The model under review builds one solid part; all positions refer to its coordinate system, in mm. A direction names the side the tool comes from. Give positions to 0.01 mm unless a question says otherwise; leave off trailing zeros. Loops run counter-clockwise (first coordinate to the right, second up) from the corner with the lowest first, then second, coordinate; pieces in that order, holes last. Notation, with made-up numbers: M 82.25,-21.75 L 103.25,-21.75 A6 cw 103.25,-12.75 Z; hole C 50,5 d4. An arc over 180 degrees is marked long. Put each result on its own line as item: value. Start each with the question number.
Autodesk Fusion 360 part; units mm, degrees
sketch "Sketch4" plane through (0, 0, 0) normal (0, 0, 1) x (1, 0, 0)
  circle A0 centre (0, 0) radius 25 construction
  dimension "d8" = 50
sketch "Sketch6" plane through (0, 0, 0) normal (1, 0, 0) x (0, 1, 0)
  line L0 (0, 0) -> (25, 0) construction
  line L1 (25, 0) -> (25, 10)
  line L2 (0, 0) -> (14.8, 0) construction
  line L3 (14.8, 0) -> (14.8, 10) construction
  line L4 (14.8, 10) -> (25, 10) construction
  line L5 (25, 10) -> (11.5, 10) construction
  line L6 (14.8, 0) -> (13.3946, 10) construction
  line L7 (14.8, 0) -> (24.8983, 0) construction
  line L8 (25, 10) -> (13.3946, 10)
  line L9 (13.3946, 10) -> (14.8, 0)
  line L10 (25, 0) -> (14.8, 0)
  dimension "d9" = 25
  dimension "d10" = 10
  dimension "d11" = 14.8
  dimension "d12" = 98
revolve "Revolve1" add sketch "Sketch6" angle 360 about axis through (0, 0, 1.75) along (0, 0, 1)
sketch "Sketch7" plane through (0, 0, 0) normal (0, 0, -1) x (1, 0, 0)
  circle A0 centre (0, 0) radius 25
  circle A1 centre (0, 0) radius 14.8
extrude "Extrude3" add 1 faces at (1.9773, 21.4518, 0) along direction (0, 0, -1) blind 10
sketch "Sketch8" plane through (0, 0, -10) normal (0, 0, -1) x (1, 0, 0)
  circle A0 centre (0, 0) radius 25
  circle A1 centre (0, 0) radius 14.8
  circle A2 centre (0, 0) radius 14.8
  circle A3 centre (0, 0) radius 25
  line L0 (1.5, 14.7238) -> (1.5, 24.955)
  line L1 (-1.5, 14.7238) -> (-1.5, 24.955)
  line L2 (-14.7238, 1.5) -> (-24.955, 1.5)
  line L3 (-14.7238, -1.5) -> (-24.955, -1.5)
  line L4 (-1.5, -14.7238) -> (-1.5, -24.955)
  line L5 (1.5, -14.7238) -> (1.5, -24.955)
  line L6 (14.7238, -1.5) -> (24.955, -1.5)
  line L7 (14.7238, 1.5) -> (24.955, 1.5)
  dimension "d19" = 360
extrude "Extrude4" add sketch "Sketch8" along normal blind 15 contours A0 A1 A2 A3 L0 L7 | A0 A1 A2 A3 L5 L6 | A0 A1 A2 A3 L1 L2 | A0 A1 A2 A3 L3 L4
Item 1: Consider section C-C, the plane x = 20. Write out the cut boundary in (y, z).
Item 2: Consider section A-A, the plane x = 0. Write out the cut boundary in (y, z).
Item 3: Draft analysis for pull direction X (two halves, no side actions). For faces 4 (the flat face through (11, 11, 10)), 5 (the flat face through (0, -20, -10)), 6 (the flat face through (0, 20, -10)), state which applies: +X half, -X half, draft (parallel to the pull), parting line (faces both ways), or undercut.
Item 4: To check wall thickness, follow L1, parallel to X at y = 0, z = -6; L2, parallel to X at y = -1.5, z = -4. State the ranges of each line that lie inside material, in increasing order. Write a range as [from, to].
Item 5: Tool access review of faces 1 (the flat face through (-20, 1.5, -17)), 2 (the flat face through (1.5, 20, -17)), 3 (the conical face through (-13.467, -2.99, 7.152)): name each direction out of +Z, -Z, +X, -X, +Y, -Y from which nothing blocks a thin tool from reaching the whole face with its end or side.
Item 6: Clearance check with flat-ended pins moving along their axes: pin 1 Ø8 at (y, z) = (18.5, -20) entering from +X; pin 2 Ø1 at (y, z) = (-3, -19.5) entering from -X; pin 3 Ø2 at (x, z) = (8.5, -5.5) entering from -Y. State where each tip first meets the part, or that it passes through.
Item 7: Consider section B-B, the plane z = -19. Write out the cut boundary in (x, y) (3 decimals).
Report:
1. outline: M -15,-25 L -1.5,-25 L -1.5,-10 L 1.5,-10 L 1.5,-25 L 15,-25 L 15,10 L -15,10 Z
2. outline: M -25,-10 L -14.8,-10 L -14.8,0 L -13.39,10 L -25,10 Z; M 13.39,10 L 14.8,0 L 14.8,-10 L 25,-10 L 25,10 Z
3. face 4: draft
3. face 5: undercut
3. face 6: undercut
4. L1: [-25, -14.8], [14.8, 25]
4. L2: [-24.95, -14.72], [14.72, 24.95]
5. face 1: -Z, +X, -X
5. face 2: -Z, +Y, -Y
5. face 3: -Z
6. pin 1: x = 20.37
6. pin 2: x = -24.87
6. pin 3: y = -23.85
7. outline: M -24.955,-1.5 A25 ccw -1.5,-24.955 L -1.5,-14.724 A14.8 cw -14.724,-1.5 Z; M -24.955,1.5 L -14.724,1.5 A14.8 cw -1.5,14.724 L -1.5,24.955 A25 ccw Z; M 1.5,-24.955 A25 ccw 24.955,-1.5 L 14.724,-1.5 A14.8 cw 1.5,-14.724 Z; M 1.5,14.724 A14.8 cw 14.724,1.5 L 24.955,1.5 A25 ccw 1.5,24.955 Z
